from build123d import *

# Parameters (mm, degrees)
SKETCH1_W           = 41.275
SKETCH1_H           = 85.725
BOSS_EXTRUDE1_DEPTH = 0.79375
SKETCH2_W           = 34.925
SKETCH2_H           = 9.525
BOSS_EXTRUDE2_DEPTH = 6.35
BOSS_EXTRUDE3_DEPTH = 19.05
SKETCH4_W           = 11.1125
SKETCH4_H           = 11.1125
BOSS_EXTRUDE4_DEPTH = 6.35
SKETCH5_R           = 2.38125
BOSS_EXTRUDE5_DEPTH = 3.175
SKETCH6_W           = 4.7625
SKETCH6_H           = 19.05
BOSS_EXTRUDE6_DEPTH = 19.05
SKETCH7_W           = 11.1125
SKETCH7_H           = 14.2875
BOSS_EXTRUDE7_DEPTH = 22.225
SKETCH8_R           = 1.5875
CUT_EXTRUDE1_DEPTH  = 53.507627422


with BuildPart() as part:
    # Sketch1 → Boss-Extrude1 (new body)
    with BuildSketch(Plane(origin=(0, 0, 0), x_dir=(1, 0, 0), z_dir=(0, 1, 0))):
        Rectangle(SKETCH1_W, SKETCH1_H)
    extrude(amount=BOSS_EXTRUDE1_DEPTH)

    # Sketch2 → Boss-Extrude2 (add)
    with BuildSketch(Plane(origin=(0, 0.79375, 0), x_dir=(1, 0, 0), z_dir=(0, 1, 0))):
        with Locations((-3.175, -25.4)):
            Rectangle(SKETCH2_W, SKETCH2_H)
    extrude(amount=BOSS_EXTRUDE2_DEPTH)

    # Sketch3 → Boss-Extrude3 (add)
    with BuildSketch(Plane(origin=(0, 0.79375, 0), x_dir=(1, 0, 0), z_dir=(0, 1, 0))):
        Polygon((14.2875, -20.6375), (14.2875, 4.7625), (-3.175, 4.7625), (-3.175, 3.175), (-17.4625, 3.175), (-17.4625, -15.875), (1.5875, -15.875), (1.5875, -20.6375), align=None)
    extrude(amount=BOSS_EXTRUDE3_DEPTH)

    # Sketch4 → Boss-Extrude4 (add)
    with BuildSketch(Plane(origin=(0, 0.79375, 0), x_dir=(1, 0, 0), z_dir=(0, 1, 0))):
        with Locations((-8.73125, 15.08125)):
            Rectangle(SKETCH4_W, SKETCH4_H)
    extrude(amount=BOSS_EXTRUDE4_DEPTH)

    # Sketch5 → Boss-Extrude5 (add)
    with BuildSketch(Plane(origin=(0, 7.14375, 0), x_dir=(1, 0, 0), z_dir=(0, 1, 0))):
        with Locations(Location((-8.73125, 15.08125, 0), (0, 0, 270))):
            Circle(SKETCH5_R)
    extrude(amount=BOSS_EXTRUDE5_DEPTH)

    # Sketch6 → Boss-Extrude6 (add)
    with BuildSketch(Plane(origin=(0, 0.79375, 0), x_dir=(1, 0, 0), z_dir=(0, 1, 0))):
        with Locations((-0.79375, 15.875)):
            Rectangle(SKETCH6_W, SKETCH6_H)
    extrude(amount=BOSS_EXTRUDE6_DEPTH)

    # Sketch7 → Boss-Extrude7 (add)
    with BuildSketch(Plane(origin=(0, 0.79375, 0), x_dir=(1, 0, 0), z_dir=(0, 1, 0))):
        with Locations((-3.96875, 32.54375)):
            Rectangle(SKETCH7_W, SKETCH7_H)
    extrude(amount=BOSS_EXTRUDE7_DEPTH)

    # Sketch8 → Cut-Extrude1 (cut, through all)
    with BuildSketch(Plane(origin=(0, 0.79375, 0), x_dir=(1, 0, 0), z_dir=(0, 1, 0))):
        with Locations(Location((-17.4625, 39.6875, 0), (0, 0, 270))):
            Circle(SKETCH8_R)
        with Locations(Location((17.4625, 39.6875, 0), (0, 0, 270))):
            Circle(SKETCH8_R)
        with Locations(Location((-17.4625, -39.6875, 0), (0, 0, 270))):
            Circle(SKETCH8_R)
        with Locations(Location((17.4625, -39.6875, 0), (0, 0, 270))):
            Circle(SKETCH8_R)
    extrude(amount=-CUT_EXTRUDE1_DEPTH, mode=Mode.SUBTRACT)


solid = part.part
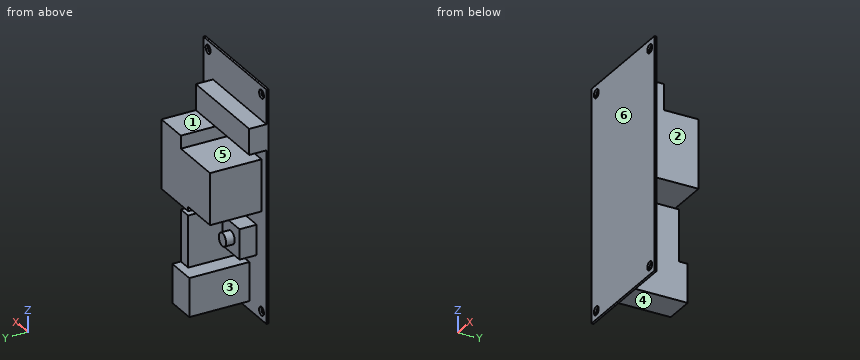
Input: part model. Units: mm. Frame: model coordinates. Face numbers are marked on the shaded views. A direction names the side the tool comes from. Round coordinates to 2 decimals unless told otherwise and drop trailing zeros. Order: outer loops, then holes, each group sorted by start corner. A loop starts at its lowest first (then second) coordinate and runs counter-clockwise, first axis right, second up. Notation, with made-up numbers: (-12, 70.5) - (-5, 70.5) arc R19 cw to (-5, 75.5) - close; hole circle Ø5 at (84, 31). An arc over 180 degrees is marked (long way). Answer as a JSON object with one key per item and string values. Group by question number.
(1) Pin query (flat end, axial travel): P1, Ø9, axis at x = -2.5, y = 16.5, coming from the -Z side; P2, Ø3, axis at y = 15.5, z = 10, coming from the -X side; P3, Ø5, axis at x = 5, y = 6.5, coming from the -Z side. Return the tip coordinate at first contact, or that it passes through.
(2) Reachability of the marked faces 1, 2 and 3 from +Z, -Z, +X, -X, +Y, -Y: full face, straight path, thin tool, end or side. Return the list, or none.
(3) Cut plane C-C (z = -32.5). Return loops of the section in (x, y) (1 decimal).
(4) Draft query along Z for the marked faces 4, 5 and 6. Return one class per face: released by +Z, released by -Z, zero draft, split by the parting line, or undercut.
(5) Material intervals for probe 1 along Z at (x, y) = (-9, 5.25) (1 decimal); probe 2 along Z at (x, y) = (-11.5, 5.5) (1 decimal); probe 3 along Z at (x, y) = (-9, 7.5) (1 decimal), sorted ascending. Write a range as from..to.
(6) Cut plane B-B (x = -12). Return loops of the section in (y, z) (1 decimal), then the cut area to 3 significant figures.
(7) Cut plane D-D (y = 8.75). Count the separate pieces of the cut face and the enclosed holes in it, then the cut area to 3 significant figures.
Here are the results:
{
 "1": {"P1": "stops at z = -39.69", "P2": "stops at x = -17.46", "P3": "stops at z = -4.76"},
 "2": {"face 1": "+Z, +X, -X, +Y", "face 2": "+Z, -Z, +X, +Y", "face 3": "-Z, -X, +Y"},
 "3": {"outline": "(-20.6, 0) - (20.6, 0) - (20.6, 0.8) - (1.6, 0.8) - (1.6, 23) - (-9.5, 23) - (-9.5, 0.8) - (-20.6, 0.8) - close"},
 "4": {"face 4": "released by -Z", "face 5": "undercut", "face 6": "zero draft"},
 "5": {"probe 1": "z = -39.7..-25.4, -20.6..-9.5, -3.2..15.9, 20.6..30.2", "probe 2": "z = -20.6..-9.5, -3.2..15.9, 20.6..30.2", "probe 3": "z = -39.7..-25.4, -17.4..-12.7, -3.2..15.9"},
 "6": {"outline": "(0, -42.9) - (0.8, -42.9) - (0.8, -20.6) - (7.1, -20.6) - (7.1, -9.5) - (0.8, -9.5) - (0.8, -3.2) - (19.8, -3.2) - (19.8, 15.9) - (0.8, 15.9) - (0.8, 20.6) - (7.1, 20.6) - (7.1, 30.2) - (0.8, 30.2) - (0.8, 42.9) - (0, 42.9) - close", "area": "562 mm^2"},
 "7": {"separate pieces": "3", "enclosed holes": "0", "area": "960 mm^2"}
}
